Check sheet for the drawn part. Datum: minimum x, y, z corner. Units: mm. A direction names the side the tool comes from. Give positions to 0.01 mm unless a question says otherwise; leave off trailing zeros. Loops run counter-clockwise (first coordinate to the right, second up) from the corner with the lowest first, then second, coordinate; pieces in that order, holes last.
1. Go/stop test with flat-tipped pins: pin 1 Ø1.9 at (y, z) = (60.5, 2) entering from -X; pin 2 Ø0.9 at (x, z) = (29.5, 3.5) entering from -Y; pin 3 Ø3 at (x, z) = (24.5, 4) entering from +Y. Record where each tip stops, or that it passes through.
2. Cross-section at D-D, the plane x = 15.5. Record the cut outline in (y, z).
3. Cross-section at A-A, the plane y = 31.75. Record the cut outline in (x, z), plus the area to 3 significant figures.
4. Tool access check on the marked faces 1, 2, 3, 4 and 5. Record the directions out of +Z, -Z, +X, -X, +Y, -Y that give a thin tool (end or side, any length) a straight path to the whole face; none if there is none.
5. Release check for a two-part mould opening along Y. For the marked faces 6, 7 and 8 record: +Y half, -Y half, draft (parallel to the pull), parting line (faces both ways), or undercut.
6. Material ranges on L1, parallel to X at y = 32, z = 4.75; L2, parallel to Y at x = 17, z = 2.75; L3, parallel to Y at x = 12, z = 1.5, recorded low to high.
7. Cross-section at C-C, the plane x = 8. Record the cut outline in (y, z), plus the area to 3 significant figures.
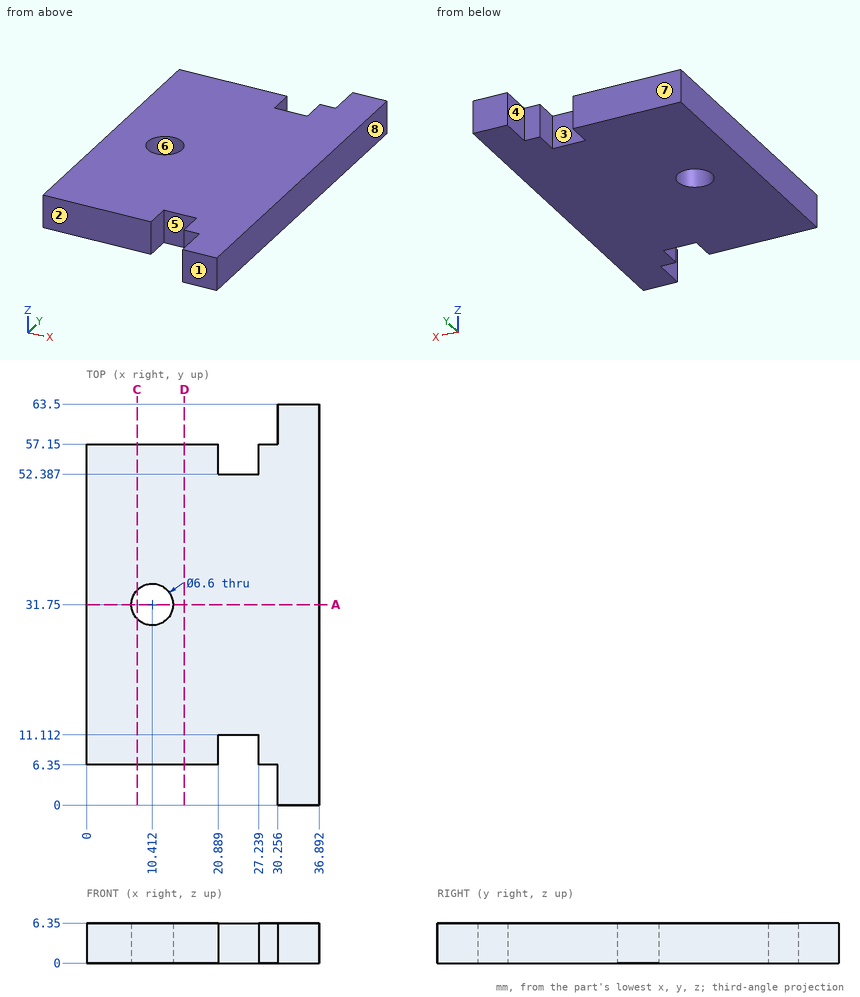
Result:
1. pin 1: stops at x = 30.26
1. pin 2: stops at y = 6.35
1. pin 3: stops at y = 52.39
2. outline: (6.35, 0) - (57.15, 0) - (57.15, 6.35) - (6.35, 6.35) - close
3. outline: (0, 0) - (7.11, 0) - (7.11, 6.35) - (0, 6.35) - close; (13.71, 0) - (36.89, 0) - (36.89, 6.35) - (13.71, 6.35) - close
3. area: 192 mm2
4. face 1: +Z, -Z, +X, -X, -Y
4. face 2: +Z, -Z, -X, -Y
4. face 3: +Z, -Z, +Y
4. face 4: +Z, -Z, -X, +Y
4. face 5: +Z, -Z, -Y
5. face 6: undercut
5. face 7: +Y half
5. face 8: draft
6. L1: x = 0 to 7.12, 13.7 to 36.89
6. L2: y = 6.35 to 57.15
6. L3: y = 6.35 to 28.86, 34.64 to 57.15
7. outline: (6.35, 0) - (29.5, 0) - (29.5, 6.35) - (6.35, 6.35) - close; (34, 0) - (57.15, 0) - (57.15, 6.35) - (34, 6.35) - close
7. area: 294 mm2
